Autodesk Inventor part; units mm, degrees
ref_plane "YZ Plane" through (0, 0, 0) normal (1, 0, 0) x (0, 1, 0)
ref_plane "XZ Plane" through (0, 0, 0) normal (0, 1, 0) x (-1, 0, 0)
ref_plane "XY Plane" through (0, 0, 0) normal (0, 0, 1) x (1, 0, 0)
sketch "Sketch1" plane through (0, 0, 0) normal (1, 0, 0) x (0, 1, 0)
  line L0 (-7.5, -7.5) -> (7.5, -7.5)
  line L1 (7.5, -7.5) -> (7.5, 7.5)
  line L2 (7.5, 7.5) -> (-7.5, 7.5)
  line L3 (-7.5, 7.5) -> (-7.5, -7.5)
  line L4 (-7.5, -7.5) -> (7.5, 7.5) construction
  line L5 (7.5, -7.5) -> (-7.5, 7.5) construction
  line L6 (7.5, 1.5) -> (4.5, 1.5)
  line L7 (4.5, 1.5) -> (4.5, -1.5)
  line L8 (4.5, -1.5) -> (7.5, -1.5)
  line L9 (7.5, -1.5) -> (7.5, 1.5)
  line L10 (1.5, 7.5) -> (-1.5, 7.5)
  line L11 (-1.5, 7.5) -> (-1.5, 4.5)
  line L12 (-1.5, 4.5) -> (1.5, 4.5)
  line L13 (1.5, 4.5) -> (1.5, 7.5)
  line L14 (-7.5, 1.5) -> (-4.5, 1.5)
  line L15 (-4.5, 1.5) -> (-4.5, -1.5)
  line L16 (-4.5, -1.5) -> (-7.5, -1.5)
  line L17 (-7.5, -1.5) -> (-7.5, 1.5)
  line L18 (-1.5, -7.5) -> (1.5, -7.5)
  line L19 (1.5, -7.5) -> (1.5, -4.5)
  line L20 (1.5, -4.5) -> (-1.5, -4.5)
  line L21 (-1.5, -4.5) -> (-1.5, -7.5)
  point P0 (0, 0)
  dimension "d0" = 15
  dimension "d1" = 3
  dimension "d2" = 3
  dimension "d3" = 1.5
  dimension "d4" = 1.5
extrude "Extrusion1" add sketch "Sketch1" along normal blind 300 contours L3 L16 L15 L14 L2 L11 L12 L13 L1 L6 L7 L8 L0 L19 L20 L21
properties part number "Beam_300mm" material "Aluminum 6061"
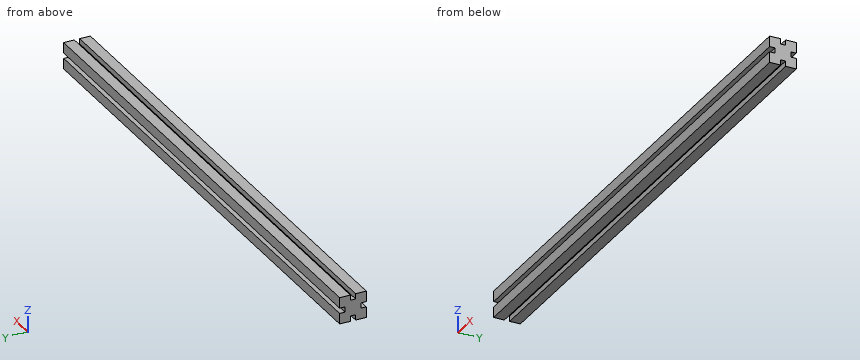
Source: CAD feature listing. Evaluate the final solid. Frame: model axes, mm. Give positions to 0.01 mm unless a question says otherwise; leave off trailing zeros. Loops run counter-clockwise (first coordinate to the right, second up) from the corner with the lowest first, then second, coordinate; pieces in that order, holes last. Notation, with made-up numbers: (76, 16) -> (127, 16) arc R17 cw to (127, 23) -> close; hole circle Ø7 at (21, 2). An arc over 180 degrees is marked (long way). Use a Markdown table: item, result. Add a question column.
1) Section query A-A, the plane x = 231.5. Return the cut outline in (y, z).
2) First-contact query: pin 1 (1 mm diameter, centred on x = 173, z = 0.5, fed in from -Y); pin 2 (1.5 mm diameter, centred on x = 90.5, y = -0.5, fed in from -Z); pin 3 (1.5 mm diameter, centred on x = 162.5, z = 0, fed in from +Y). Flat tips, straight axial feed; report the tip coordinate or a pass-through.
3) Line query: line 1 along Y through (x, z) = (267.5, -5.25); line 2 along Y through (x, z) = (124, -0.75). Output: solid intervals per line, ascending. Write a range as [from, to].
Numbers:
| question | item | result |
|---|---|---|
| 1 | outline | (-7.5, -7.5) -> (-1.5, -7.5) -> (-1.5, -4.5) -> (1.5, -4.5) -> (1.5, -7.5) -> (7.5, -7.5) -> (7.5, -1.5) -> (4.5, -1.5) -> (4.5, 1.5) -> (7.5, 1.5) -> (7.5, 7.5) -> (1.5, 7.5) -> (1.5, 4.5) -> (-1.5, 4.5) -> (-1.5, 7.5) -> (-7.5, 7.5) -> (-7.5, 1.5) -> (-4.5, 1.5) -> (-4.5, -1.5) -> (-7.5, -1.5) -> close |
| 2 | pin 1 | stops at y = -4.5 |
| 2 | pin 2 | stops at z = -4.5 |
| 2 | pin 3 | stops at y = 4.5 |
| 3 | line 1 | y = [-7.5, -1.5], [1.5, 7.5] |
| 3 | line 2 | y = [-4.5, 4.5] |
